from build123d import *

# Parameters (mm, degrees)
SKETCH_1_R          = 2
EXTRUDE_1_DEPTH     = 20.5
SKETCH_2_R          = 2
CUT_EXTRUDE_1_DEPTH = 20.5
MOVE_BODY_1_ANGLE   = 90


with BuildPart() as part:
    # 草图1 → 凸台-拉伸1 (new body)
    with BuildSketch(Plane(origin=(0, 0, 0), x_dir=(0, 0, -1), z_dir=(1, 0, 0))):
        with BuildLine():
            Line((-7, 18), (7, 18))
            Line((7, 18), (7, 14))
            ThreePointArc((7, 14), (8.171572875, 11.171572875), (11, 10))
            Line((11, 10), (19, 10))
            Line((19, 10), (19, 0))
            Line((19, 0), (7, 0))
            Line((7, 0), (-7, 0))
            Line((-7, 0), (-19, 0))
            Line((-19, 0), (-19, 10))
            Line((-19, 10), (-11, 10))
            ThreePointArc((-11, 10), (-8.171572875, 11.171572875), (-7, 14))
            Line((-7, 14), (-7, 18))
        make_face()
        with Locations((0, 13)):
            Circle(SKETCH_1_R, mode=Mode.SUBTRACT)
        with Locations((0, 7)):
            Circle(SKETCH_1_R, mode=Mode.SUBTRACT)
    extrude(amount=EXTRUDE_1_DEPTH)

    # 草图2 → 切除-拉伸1 (cut)
    with BuildSketch(Plane(origin=(0, 10, 0), x_dir=(1, 0, 0), z_dir=(0, 1, 0))):
        with Locations(Location((10.25, 14, 0), (0, 0, 270))):
            Circle(SKETCH_2_R)
        with Locations(Location((10.25, -14, 0), (0, 0, 270))):
            Circle(SKETCH_2_R)
    extrude(amount=-CUT_EXTRUDE_1_DEPTH, mode=Mode.SUBTRACT)


with BuildPart() as part_1:
    # Move Body 1: moved
    add(part.part.rotate(Axis((10.25, 0, 0), (0, -1, 0)), MOVE_BODY_1_ANGLE))


solid = part_1.part
For this review, take the finished solid that the model builds, in its own axes (mm). A direction names the side the tool comes from. Round coordinates to 2 decimals unless told otherwise and drop trailing zeros. Write each loop counter-clockwise with the first axis right and the second up, starting at its lowest first coordinate (ties: lowest second). Pieces come first, ordered by that corner, then holes. Notation, with made-up numbers: M 73.5,67.25 L 80.5,67.25 A22 ccw 80.5,102.25 Z; hole C 2,46.25 d6. An arc over 180 degrees is marked long. Write item = value, one per line. Start each with the question number.
(1) We need section A-A (y = 7). Give the boundary of the cut face in (x, z).
(2) The part is to be moulded in two halves that separate along Z. For faces 4 (the face through (8.776, 8.352, -0.143)), 5 (the face through (-2.163, 5.07, -1.217)), 6 (the face through (11, 3, -10.25)), 7 (the face through (26.248, 5.07, 0.088)), say which applies: +Z half, -Z half, draft (parallel to the pull), parting line (faces both ways), or undercut.
(3) Clearance check with flat-ended pins moving along their axes: pin 1 Ø2.5 at (x, z) = (24.25, 0) entering from +Y; pin 2 Ø10 at (x, z) = (-2.5, -5.5) entering from +Y; pin 3 Ø1.2 at (y, z) = (15.5, 0.5) entering from +X; pin 4 Ø3 at (y, z) = (14.5, 6.5) entering from +X. State where each tip first meets the part, or that it passes through.
(4) We need section C-C (z = -3.75). Give the boundary of the cut face in (x, y), then the cut area to 3 significant figures.
(5) For faces 1 (the face through (3.25, 16, 0)), 2 (the face through (11, 3, 10.25)), 3 (the face through (17.25, 16, 0)), list the 3-axis set-ups (+Z, -Z, +X, -X, +Y, -Y) from which the entire face can be reached by the end or side of a thin tool; tool diameter is ignored.
(6) For line 1 along Y through (x, z) = (10.25, 2); line 2 along Y through (x, z) = (12, 4.75); line 3 along X through (y, z) = (8.5, -9.5), list the stretches that pass through material, from the lowest coordinate up.
(7) We need section D-D (z = -0.5). Give the boundary of the cut face in (x, y), then the cut area to 3 significant figures.
(8) We need section B-B (x = 10.25). Give the boundary of the cut face in (y, z).
Results found:
q1.outline = M -8.75,-10.25 L 8.25,-10.25 L 8.25,10.25 L -8.75,10.25 Z; M 12.25,-10.25 L 29.25,-10.25 L 29.25,10.25 L 12.25,10.25 Z; hole C -3.75,0 d4; hole C 24.25,0 d4
q2.face_4 = draft
q2.face_5 = undercut
q2.face_6 = -Z half
q2.face_7 = undercut
q3.pin_1 = through
q3.pin_2 = 11.67
q3.pin_3 = 17.25
q3.pin_4 = 17.38
q4.outline = M -8.75,0 L 29.25,0 L 29.25,10 L 21.25,10 A4 cw 17.25,14 L 17.25,18 L 3.25,18 L 3.25,14 A4 cw -0.75,10 L -8.75,10 Z; hole C 10.25,7 d4; hole C 10.25,13 d4
q4.area = 474 mm²
q5.face_1 = +Z, -Z, -X, +Y
q5.face_2 = +Z, +X, -X, +Y, -Y
q5.face_3 = +Z, -Z, +X, +Y
q6.line_1 = 0 to 5, 9 to 11, 15 to 18
q6.line_2 = 0 to 6.03, 7.97 to 12.03, 13.97 to 18
q6.line_3 = -8.75 to 8.93, 11.57 to 29.25
q7.outline = M -8.75,0 L -5.69,0 L -5.69,10 L -8.75,10 Z; M -1.81,0 L 22.31,0 L 22.31,10 L 21.25,10 A4 cw 17.25,14 L 17.25,18 L 3.25,18 L 3.25,14 A4 cw -0.75,10 L -1.81,10 Z; M 26.19,0 L 29.25,0 L 29.25,10 L 26.19,10 Z; hole C 10.25,7 d4; hole C 10.25,13 d4
q7.area = 396 mm²
q8.outline = M 0,-10.25 L 5,-10.25 L 5,10.25 L 0,10.25 Z; M 9,-10.25 L 11,-10.25 L 11,10.25 L 9,10.25 Z; M 15,-10.25 L 18,-10.25 L 18,10.25 L 15,10.25 Z
